```python
from build123d import *

# Parameters (mm, degrees)
SALIENTE_EXTRUIR1_DEPTH = 175.8
CROQUIS3_W              = 20
CROQUIS3_H              = 3
SALIENTE_EXTRUIR2_DEPTH = 175.8
CROQUIS4_W              = 74.9
CROQUIS4_H              = 20
CROQUIS4_R              = 2.5
CORTAR_EXTRUIR1_DEPTH   = 165.8
SALIENTE_EXTRUIR3_START = -26
SALIENTE_EXTRUIR3_DEPTH = 26
CORTAR_EXTRUIR2_DEPTH   = 26


with BuildPart() as part:
    # Croquis2 → Saliente-Extruir1 (new body)
    with BuildSketch(Plane(origin=(0, 0, 0), x_dir=(0, 0, -1), z_dir=(1, 0, 0))):
        Polygon((0, 27.28), (0, 30.28), (-90.45, 3), (-90.45, 0), align=None)
    extrude(amount=SALIENTE_EXTRUIR1_DEPTH)

    # Croquis3 → Saliente-Extruir2 (add)
    with BuildSketch(Plane(origin=(175.8, 0, 0), x_dir=(0, 0, -1), z_dir=(1, 0, 0))):
        with Locations((10, 28.78)):
            Rectangle(CROQUIS3_W, CROQUIS3_H)
    extrude(amount=-SALIENTE_EXTRUIR2_DEPTH)

    # Croquis4 → Cortar-Extruir1 (cut)
    with BuildSketch(Plane(origin=(0, 30.28, 0), x_dir=(1, 0, 0), z_dir=(0, 1, 0))):
        with Locations((138.35, 10)):
            Rectangle(CROQUIS4_W, CROQUIS4_H)
        with Locations((37.45, 10)):
            Rectangle(CROQUIS4_W, CROQUIS4_H)
        with Locations((87.9, 10)):
            Circle(CROQUIS4_R)
    extrude(amount=-CORTAR_EXTRUIR1_DEPTH, mode=Mode.SUBTRACT)

    # Croquis5 → Saliente-Extruir3 (add)
    with BuildSketch(Plane(origin=(100.9, 0, 0), x_dir=(0, 0, -1), z_dir=(1, 0, 0)).offset(SALIENTE_EXTRUIR3_START)):
        Polygon((1.878378592, 30.28), (0.745913837, 36.00039966), (-0.555574899, 29.798151404), align=None)
    extrude(amount=SALIENTE_EXTRUIR3_DEPTH)

    # Croquis6 → Cortar-Extruir2 (cut)
    with BuildSketch(Plane(origin=(100.9, 0, 0), x_dir=(0, 0, -1), z_dir=(1, 0, 0))):
        Polygon((0.130372487, 33.067035615), (1.312146214, 33.14019983), (0.745913837, 36.00039966), align=None)
    extrude(amount=-CORTAR_EXTRUIR2_DEPTH, mode=Mode.SUBTRACT)


solid = part.part
```
The model under review builds one solid part; all positions refer to its coordinate system, in mm. A direction names the side the tool comes from. Give positions to 0.01 mm unless a question says otherwise; leave off trailing zeros. Write each loop counter-clockwise with the first axis right and the second up, starting at its lowest first coordinate (ties: lowest second). Pieces come first, ordered by that corner, then holes. Notation, with made-up numbers: M 3,33 L 39,33 A27 cw 39,52 Z; hole C 10.5,48.5 d10. An arc over 180 degrees is marked long. Answer in a Markdown table with one row per item.
Item 1: Draft analysis for pull direction X (two halves, no side actions). For faces 3 (the face through (91, 27.28, -10)), 4 (the face through (85.4, 28.8, -10.1)), 5 (the face through (175.8, 15, 45)), state which applies: +X half, -X half, draft (parallel to the pull), parting line (faces both ways), or undercut.
Check sheet entries:
| item | result |
|---|---|
| face 3 | draft |
| face 4 | undercut |
| face 5 | +X half |
Item 2: Add section D-D on y = 24.5. Give the boundary of the cut face in (x, z).
Check sheet entries:
| item | result |
|---|---|
| outline | M 0,9.22 L 175.8,9.22 L 175.8,19.16 L 0,19.16 Z |
Item 3: Add section A-A on z = -10. Give the boundary of the cut face in (x, y).
Check sheet entries:
| item | result |
|---|---|
| outline | M 74.9,27.28 L 85.4,27.28 L 85.4,30.28 L 74.9,30.28 Z; M 90.4,27.28 L 100.9,27.28 L 100.9,30.28 L 90.4,30.28 Z |
Item 4: For line 1 along X through (y, z) = (28, -10); line 2 along Y through (x, z) = (126, 72); line 3 along Y through (x, z) = (77.5, 53.5), list the stretches that pass through material, from the lowest coordinate up.
Check sheet entries:
| item | result |
|---|---|
| line 1 | 74.9 to 85.4, 90.4 to 100.9 |
| line 2 | 5.56 to 8.56 |
| line 3 | 11.14 to 14.14 |
Item 5: Add section C-C on x = 23.5. Give the boundary of the cut face in (y, z), plus the area to 3 significant figures.
Check sheet entries:
| item | result |
|---|---|
| outline | M 0,90.45 L 27.28,0 L 30.28,0 L 3,90.45 Z |
| area | 271 mm2 |
Item 6: For P1, Ø4, axis at x = 121, z = 39, coming from the -Y side; P2, Ø0.9, axis at x = 22.5, y = 29, coming from the -Z side; P3, Ø3, axis at x = 107.5, z = 60.5, coming from the +Y side; P4, Ø8, axis at x = 69, z = -7.5, coming from the +Y side, all flat-tipped, find the tip position at first contact; note any pin that passes through.
Check sheet entries:
| item | result |
|---|---|
| P1 | y = 14.91 |
| P2 | z = 0 |
| P3 | y = 12.49 |
| P4 | through |
Item 7: Tool access review of faces 1 (the face through (88, 30.28, -13)), 2 (the face through (86.67, 13.45, 45.86)): name each direction out of +Z, -Z, +X, -X, +Y, -Y from which nothing blocks a thin tool from reaching the whole face with its end or side.
Check sheet entries:
| item | result |
|---|---|
| face 1 | -Z, +X, -X, +Y |
| face 2 | -Z, +X, -X, -Y |
Item 8: Add section B-B on x = 87.9. Give the boundary of the cut face in (y, z).
Check sheet entries:
| item | result |
|---|---|
| outline | M 0,90.45 L 27.28,0 L 27.28,-7.5 L 30.28,-7.5 L 30.28,-1.88 L 33.14,-1.31 L 33.07,-0.13 L 30.13,0.49 L 3,90.45 Z; M 27.28,-20 L 30.28,-20 L 30.28,-12.5 L 27.28,-12.5 Z |
